Autodesk Inventor part; units mm, degrees
ref_plane "YZ Plane" through (0, 0, 0) normal (1, 0, 0) x (0, 1, 0)
ref_plane "XZ Plane" through (0, 0, 0) normal (0, 1, 0) x (-1, 0, 0)
ref_plane "XY Plane" through (0, 0, 0) normal (0, 0, 1) x (1, 0, 0)
sketch "Sketch1" plane through (0, 0, 0) normal (0, 0, 1) x (1, 0, 0)
  line L0 (0, 0) -> (0, 12.7)
  line L1 (0, 12.7) -> (12.7, 12.7)
  line L2 (12.7, 12.7) -> (12.7, 11.43)
  line L3 (12.7, 11.43) -> (1.27, 11.43)
  line L4 (1.27, 11.43) -> (1.27, 0)
  line L5 (1.27, 0) -> (0, 0)
  dimension "d0" = 12.7
  dimension "d1" = 12.7
  dimension "d2" = 1.27
  dimension "d3" = 11.43
extrude "Extrusion1" add sketch "Sketch1" along normal blind 228.6
sketch "Sketch2" plane through (0, 12.7, 0) normal (0, 1, 0) x (1, 0, 0)
  line L0 (0, 0) -> (12.7, 0)
  line L1 (12.7, -228.6) -> (0, -228.6)
  line L2 (12.7, 0) -> (12.7, -228.6)
  line L3 (0, -228.6) -> (12.7, -215.9)
  line L4 (0, 0) -> (12.7, -12.7)
  dimension "d6" = 45
  dimension "d7" = 45
extrude "Extrusion2" cut sketch "Sketch2" against normal blind 228.6
properties part number "Aluminum Angle 2" material "Aluminum 6061"
Check sheet for the modelled part. Datum: model origin and axes. Units: mm. A direction names the side the tool comes from. Coordinates: 2 decimals unless noted, no trailing zeros. Write each loop counter-clockwise with the first axis right and the second up, starting at its lowest first coordinate (ties: lowest second). Pieces come first, ordered by that corner, then holes. Notation, with made-up numbers: (49.25, 51) -> (74.25, 51) arc R21 ccw to (74.25, 80) -> close; hole circle Ø4 at (35, -37). An arc over 180 degrees is marked (long way). Use a Markdown table: item, result.
1. Tool access check on faces 1 (the flat face through (1.27, 6, 113)), 2 (the flat face through (0, 6, 113)). Record the directions out of +Z, -Z, +X, -X, +Y, -Y that give a thin tool (end or side, any length) a straight path to the whole face; none if there is none.
Reported:
| item | result |
|---|---|
| face 1 | +Z, -Z, +X, -Y |
| face 2 | +Z, -Z, -X, +Y, -Y |
2. Sectioned sample at A-A (z = 204). Enter the section's corners in (x, y), plus the area to 3 significant figures.
Reported:
| item | result |
|---|---|
| outline | (0, 0) -> (1.27, 0) -> (1.27, 11.43) -> (12.7, 11.43) -> (12.7, 12.7) -> (0, 12.7) -> close |
| area | 30.6 mm2 |
3. Sectioned sample at B-B (x = 9.75). Enter the section's corners in (y, z).
Reported:
| item | result |
|---|---|
| outline | (11.43, 9.75) -> (12.7, 9.75) -> (12.7, 218.85) -> (11.43, 218.85) -> close |
4. Sectioned sample at C-C (y = 2). Enter the section's corners in (x, z), plus the area to 3 significant figures.
Reported:
| item | result |
|---|---|
| outline | (0, 0) -> (1.27, 1.27) -> (1.27, 227.33) -> (0, 228.6) -> close |
| area | 289 mm2 |
5. Scan lines: line 1 along Y through (x, z) = (9.5, 199); line 2 along X through (y, z) = (2.25, 196); line 3 along Z through (x, y) = (0.75, 3.75). Record each from-to range of solid material in increasing order.
Reported:
| item | result |
|---|---|
| line 1 | y = 11.43 to 12.7 |
| line 2 | x = 0 to 1.27 |
| line 3 | z = 0.75 to 227.85 |
6. Go/stop test with flat-tipped pins: pin 1 Ø4 at (x, y) = (6, 10.5) entering from +Z; pin 2 Ø5.5 at (y, z) = (4.5, 75.5) entering from +X; pin 3 Ø3.5 at (x, z) = (5, 62) entering from -Y. Record where each tip stops, or that it passes through.
Reported:
| item | result |
|---|---|
| pin 1 | stops at z = 224.37 |
| pin 2 | stops at x = 1.27 |
| pin 3 | stops at y = 11.43 |
